Here's how the part is built. I have some questions about the finished solid (model axes, mm). Face numbers are marked on the shaded views. Coordinates: 2 decimals unless noted, no trailing zeros. Write each loop counter-clockwise with the first axis right and the second up, starting at its lowest first coordinate (ties: lowest second). Pieces come first, ordered by that corner, then holes.
(1) For pin 1 Ø3 at (y, z) = (9.5, -14.5) entering from -X; pin 2 Ø3.5 at (x, z) = (2, 70) entering from +Y; pin 3 Ø1.8 at (x, z) = (55, -36) entering from +Y; pin 4 Ø1.5 at (y, z) = (3.5, -42.5) entering from +X, each with a flat end and sliding along its axis, tell me the tip position at first contact or that it passes through.
(2) Please list where these lines run through material, in increasing order: probe 1 along X at (y, z) = (2.65, -7.5); probe 2 along Z at (x, y) = (-65, 3.8); probe 3 along Z at (x, y) = (83, 3.5).
(3) Imagine slicing it at A-A, the plane z = -1.5. List the corners of the cut face in (x, y) for me.
(4) Imagine slicing it at C-C, the plane y = 2.25. State how many separate pieces and enclosed holes the cut face has, plus the area to 3 significant figures.
(5) Thinking about a two-plate mould opening in X: for the marked faces 1, 2 and 3, which applies, released by +X, released by -X, zero draft, split by the parting line, or undercut?
(6) Imagine slicing it at B-B, the plane x = -33. List the corners of the cut face in (y, z) for me.
(7) Imagine slicing it at D-D, the plane y = 18. List the corners of the cut face in (x, z) for me, plus the area to 3 significant figures.
```python
from build123d import *

# Parameters (mm, degrees)
SKETCH1_W           = 200
SKETCH1_H           = 160
BOSS_EXTRUDE1_DEPTH = 5
SKETCH2_R           = 2
CUT_EXTRUDE1_DEPTH  = 5
SKETCH3_R           = 1.5
CUT_EXTRUDE4_DEPTH  = 5
SKETCH4_R           = 1.5
CUT_EXTRUDE5_DEPTH  = 5
SKETCH5_W           = 35
SKETCH5_H           = 35
CUT_EXTRUDE6_DEPTH  = 5
SKETCH7_W           = 7
SKETCH7_H           = 40
SKETCH7_W_2         = 5
SKETCH7_W_3         = 20
SKETCH7_H_2         = 5
CUT_EXTRUDE7_DEPTH  = 5
SKETCH8_W           = 15
SKETCH8_H           = 12
SKETCH8_W_2         = 30
SKETCH8_H_2         = 6
CUT_EXTRUDE8_DEPTH  = 5
SKETCH9_W           = 20
SKETCH9_H           = 5
CUT_EXTRUDE9_DEPTH  = 5
SKETCH10_R          = 1.5
CUT_EXTRUDE10_DEPTH = 5
SKETCH11_R          = 1.5
CUT_EXTRUDE11_DEPTH = 5
SKETCH12_R          = 1.5
CUT_EXTRUDE12_DEPTH = 5
SKETCH14_W          = 2
SKETCH14_H          = 35
BOSS_EXTRUDE3_DEPTH = 20
SKETCH15_W          = 39
SKETCH15_H          = 2
BOSS_EXTRUDE4_DEPTH = 20
SKETCH16_W          = 39
SKETCH16_H          = 2
BOSS_EXTRUDE5_DEPTH = 20
SKETCH17_W          = 35
SKETCH17_H          = 18
CUT_EXTRUDE13_DEPTH = 20


with BuildPart() as part:
    # Sketch1 → Boss-Extrude1 (new body)
    with BuildSketch(Plane(origin=(0, 0, 0), x_dir=(1, 0, 0), z_dir=(0, 1, 0))):
        Rectangle(SKETCH1_W, SKETCH1_H)
    extrude(amount=BOSS_EXTRUDE1_DEPTH)

    # Sketch2 → Cut-Extrude1 (cut)
    with BuildSketch(Plane(origin=(0, 5, 0), x_dir=(1, 0, 0), z_dir=(0, 1, 0))):
        with Locations(Location((-93, 73, 0), (0, 0, 270))):
            Circle(SKETCH2_R)
        with Locations(Location((93, 73, 0), (0, 0, 90))):
            Circle(SKETCH2_R)
        with Locations(Location((93, -73, 0), (0, 0, 270))):
            Circle(SKETCH2_R)
        with Locations(Location((-93, -73, 0), (0, 0, 90))):
            Circle(SKETCH2_R)
    extrude(amount=-CUT_EXTRUDE1_DEPTH, mode=Mode.SUBTRACT)

    # Sketch3 → Cut-Extrude4 (cut)
    with BuildSketch(Plane(origin=(0, 5, 0), x_dir=(1, 0, 0), z_dir=(0, 1, 0))):
        with Locations(Location((90, 7.5, 0), (0, 0, 270))):
            Circle(SKETCH3_R)
        with Locations(Location((90, -7.5, 0), (0, 0, 90))):
            Circle(SKETCH3_R)
    extrude(amount=-CUT_EXTRUDE4_DEPTH, mode=Mode.SUBTRACT)

    # Sketch4 → Cut-Extrude5 (cut)
    with BuildSketch(Plane(origin=(0, 5, 0), x_dir=(1, 0, 0), z_dir=(0, 1, 0))):
        with Locations(Location((55, 36, 0), (0, 0, 270))):
            Circle(SKETCH4_R)
        with Locations(Location((55, -36, 0), (0, 0, 90))):
            Circle(SKETCH4_R)
    extrude(amount=-CUT_EXTRUDE5_DEPTH, mode=Mode.SUBTRACT)

    # Sketch5 → Cut-Extrude6 (cut)
    with BuildSketch(Plane(origin=(0, 5, 0), x_dir=(1, 0, 0), z_dir=(0, 1, 0))):
        with Locations((2.5, 0)):
            Rectangle(SKETCH5_W, SKETCH5_H)
    extrude(amount=-CUT_EXTRUDE6_DEPTH, mode=Mode.SUBTRACT)

    # Sketch7 → Cut-Extrude7 (cut)
    with BuildSketch(Plane(origin=(0, 5, 0), x_dir=(1, 0, 0), z_dir=(0, 1, 0))):
        with Locations((-11.5, -50)):
            Rectangle(SKETCH7_W, SKETCH7_H)
        with Locations((32.5, 0)):
            Rectangle(SKETCH7_W_2, SKETCH7_H)
        with Locations((-30, 67.5)):
            Rectangle(SKETCH7_W_3, SKETCH7_H_2)
        with Locations((-30, -67.5)):
            Rectangle(SKETCH7_W_3, SKETCH7_H_2)
    extrude(amount=-CUT_EXTRUDE7_DEPTH, mode=Mode.SUBTRACT)

    # Sketch8 → Cut-Extrude8 (cut)
    with BuildSketch(Plane(origin=(0, 5, 0), x_dir=(1, 0, 0), z_dir=(0, 1, 0))):
        with Locations((17.5, 28.5)):
            Rectangle(SKETCH8_W, SKETCH8_H)
        with Locations((85, 43)):
            Rectangle(SKETCH8_W_2, SKETCH8_H_2)
        with Locations((85, -43)):
            Rectangle(SKETCH8_W_2, SKETCH8_H_2)
    extrude(amount=-CUT_EXTRUDE8_DEPTH, mode=Mode.SUBTRACT)

    # Sketch9 → Cut-Extrude9 (cut)
    with BuildSketch(Plane(origin=(0, 5, 0), x_dir=(1, 0, 0), z_dir=(0, 1, 0))):
        with Locations((20, 67.5)):
            Rectangle(SKETCH9_W, SKETCH9_H)
    extrude(amount=-CUT_EXTRUDE9_DEPTH, mode=Mode.SUBTRACT)

    # Sketch10 → Cut-Extrude10 (cut)
    with BuildSketch(Plane(origin=(0, 5, 0), x_dir=(1, 0, 0), z_dir=(0, 1, 0))):
        with Locations(Location((-95, -25, 0), (0, 0, 270))):
            Circle(SKETCH10_R)
        with Locations(Location((-45, 68, 0), (0, 0, 270))):
            Circle(SKETCH10_R)
    extrude(amount=-CUT_EXTRUDE10_DEPTH, mode=Mode.SUBTRACT)

    # Sketch11 → Cut-Extrude11 (cut)
    with BuildSketch(Plane(origin=(0, 5, 0), x_dir=(1, 0, 0), z_dir=(0, 1, 0))):
        with Locations(Location((2, -33, 0), (0, 0, 270))):
            Circle(SKETCH11_R)
        with Locations(Location((2, -70, 0), (0, 0, 90))):
            Circle(SKETCH11_R)
        with Locations(Location((39, -70, 0), (0, 0, 270))):
            Circle(SKETCH11_R)
        with Locations(Location((39, -33, 0), (0, 0, 90))):
            Circle(SKETCH11_R)
    extrude(amount=-CUT_EXTRUDE11_DEPTH, mode=Mode.SUBTRACT)

    # Sketch12 → Cut-Extrude12 (cut)
    with BuildSketch(Plane(origin=(0, 5, 0), x_dir=(1, 0, 0), z_dir=(0, 1, 0))):
        with Locations(Location((-65, 55, 0), (0, 0, 270))):
            Circle(SKETCH12_R)
        with Locations(Location((-65, -55, 0), (0, 0, 90))):
            Circle(SKETCH12_R)
    extrude(amount=-CUT_EXTRUDE12_DEPTH, mode=Mode.SUBTRACT)

    # Sketch14 → Boss-Extrude3 (add)
    with BuildSketch(Plane(origin=(0, 5, 0), x_dir=(1, 0, 0), z_dir=(0, 1, 0))):
        with Locations((-16, 0)):
            Rectangle(SKETCH14_W, SKETCH14_H)
        with Locations((21, 0)):
            Rectangle(SKETCH14_W, SKETCH14_H)
    extrude(amount=BOSS_EXTRUDE3_DEPTH)

    # Sketch15 → Boss-Extrude4 (add)
    with BuildSketch(Plane(origin=(0, 5, 0), x_dir=(1, 0, 0), z_dir=(0, 1, 0))):
        with Locations((2.5, -18.5)):
            Rectangle(SKETCH15_W, SKETCH15_H)
    extrude(amount=BOSS_EXTRUDE4_DEPTH)

    # Sketch16 → Boss-Extrude5 (add)
    with BuildSketch(Plane(origin=(0, 5, 0), x_dir=(1, 0, 0), z_dir=(0, 1, 0))):
        with Locations((2.5, 18.5)):
            Rectangle(SKETCH16_W, SKETCH16_H)
    extrude(amount=BOSS_EXTRUDE5_DEPTH)

    # Sketch17 → Cut-Extrude13 (cut)
    with BuildSketch(Plane(origin=(22, 0, 0), x_dir=(0, 0, -1), z_dir=(1, 0, 0))):
        with Locations((0, 16)):
            Rectangle(SKETCH17_W, SKETCH17_H)
    extrude(amount=-CUT_EXTRUDE13_DEPTH, mode=Mode.SUBTRACT)


solid = part.part
```
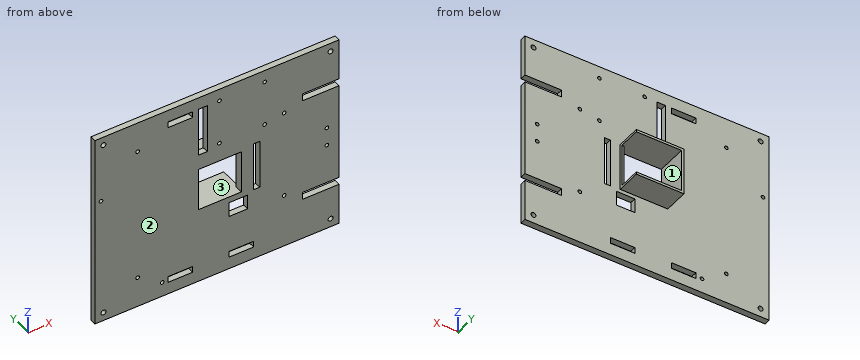
Recorded:
1. pin 1: stops at x = -17
1. pin 2: stops at y = 5
1. pin 3: passes through
1. pin 4: stops at x = 70
2. probe 1: x = -100 to -15, 20 to 30, 35 to 88.5, 91.5 to 100
2. probe 2: z = -80 to -56.5, -53.5 to 53.5, 56.5 to 80
2. probe 3: z = -80 to -46, -40 to 40, 46 to 80
3. outline: (-100, 0) - (-15, 0) - (-15, 25) - (-17, 25) - (-17, 5) - (-100, 5) - close; (20, 0) - (30, 0) - (30, 5) - (22, 5) - (22, 7) - (20, 7) - close; (35, 0) - (100, 0) - (100, 5) - (35, 5) - close
4. separate pieces: 1
4. enclosed holes: 23
4. area: 29,300 mm2
5. face 1: undercut
5. face 2: zero draft
5. face 3: undercut
6. outline: (0, -80) - (5, -80) - (5, -70) - (0, -70) - close; (0, -65) - (5, -65) - (5, 65) - (0, 65) - close; (0, 70) - (5, 70) - (5, 80) - (0, 80) - close
7. outline: (-17, -19.5) - (22, -19.5) - (22, -17.5) - (-15, -17.5) - (-15, 17.5) - (22, 17.5) - (22, 19.5) - (-17, 19.5) - close
7. area: 226 mm2
